Verification items for the finished model (mm, model axes). A direction names the side the tool comes from. Give positions to 0.01 mm unless a question says otherwise; leave off trailing zeros. Loops run counter-clockwise (first coordinate to the right, second up) from the corner with the lowest first, then second, coordinate; pieces in that order, holes last. Notation, with made-up numbers: (29.25, -19) - (55.25, -19) arc R35 cw to (55.25, 17) - close; hole circle Ø1 at (86, 35). An arc over 180 degrees is marked (long way). Put each result on its own line as item: value. Start each with the question number.
```python
from build123d import *

# Parameters (mm, degrees)
SKETCH1_W                                           = 8
SKETCH1_H                                           = 105
BASE_DEPTH                                          = 35
CSK_FOR_M4_COUNTERSUNK_FLAT_HEAD_SCREW2_D           = 4.5
CSK_FOR_M4_COUNTERSUNK_FLAT_HEAD_SCREW2_CSINK_D     = 9.4
CSK_FOR_M4_COUNTERSUNK_FLAT_HEAD_SCREW2_CSINK_ANGLE = 90
FILLET1_R                                           = 35
SKETCH8_W                                           = 8
SKETCH8_H                                           = 70
BOSS_EXTRUDE1_DEPTH                                 = 101.6
CUT_EXTRUDE1_REACH                                  = 112.968
CUT_EXTRUDE2_DEPTH                                  = 111.968463989
FILLET2_R                                           = 34.925
FILLET3_R                                           = 15.875
SKETCH12_R                                          = 12.7
CUT_EXTRUDE4_DEPTH                                  = 111.968463989
CHAMFER1_SIZE                                       = 0.396875


with BuildPart() as part:
    # Sketch1 → base (new, symmetric)
    with BuildSketch(Plane.XY):
        with Locations((4, 52.5)):
            Rectangle(SKETCH1_W, SKETCH1_H)
    extrude(amount=BASE_DEPTH, both=True)

    # CSK for M4 Countersunk Flat Head Screw2 (through all)
    with Locations(Plane.ZY):
        with Locations((-11.125, 50.730934766), (-22.25, 70), (-11.125, 89.269065234), (11.125, 89.269065234), (22.25, 70), (11.125, 50.730934766)):
            CounterSinkHole(CSK_FOR_M4_COUNTERSUNK_FLAT_HEAD_SCREW2_D / 2, CSK_FOR_M4_COUNTERSUNK_FLAT_HEAD_SCREW2_CSINK_D / 2, counter_sink_angle=CSK_FOR_M4_COUNTERSUNK_FLAT_HEAD_SCREW2_CSINK_ANGLE)

    # Fillet1
    fillet1_edges = [part.edges().sort_by_distance(p)[0] for p in [
        (4, 105, 35),
        (4, 105, -35),
    ]]
    fillet(fillet1_edges, radius=FILLET1_R - 0.0001)  # a hair under: the kernel refuses the full size

    # Sketch8 → Boss-Extrude1 (add)
    with BuildSketch(Plane.XZ):
        with Locations((4, 0)):
            Rectangle(SKETCH8_W, SKETCH8_H)
    extrude(amount=BOSS_EXTRUDE1_DEPTH)

    # Sketch9 → Cut-Extrude1 (cut, up to next)
    with BuildSketch(Plane.ZY, mode=Mode.PRIVATE) as cut_extrude1_sk1:
        with BuildLine():
            Line((2.5, 22.225), (2.5, -85.725))
            ThreePointArc((2.5, -85.725), (0, -88.225), (-2.5, -85.725))
            Line((-2.5, -85.725), (-2.5, 22.225))
            ThreePointArc((-2.5, 22.225), (0, 24.725), (2.5, 22.225))
        make_face()
    cut_extrude1_tool1 = extrude(cut_extrude1_sk1.sketch, amount=-CUT_EXTRUDE1_REACH, mode=Mode.PRIVATE) & part.part
    add(cut_extrude1_tool1.solids().sort_by_distance((0, -31.75, 0))[0], mode=Mode.SUBTRACT)

    # Sketch10 → Cut-Extrude2 (cut, through all)
    with BuildSketch(Plane(origin=(8, 0, 0), x_dir=(0, 0, -1), z_dir=(1, 0, 0))):
        with BuildLine():
            Line((15.875, 38.807302537), (15.875, -101.6))
            Line((15.875, -101.6), (35, -101.6))
            Line((35, -101.6), (35, 70))
            ThreePointArc((35, 70), (29.838104833, 51.705533624), (15.875, 38.807302537))
        make_face()
        with BuildLine():
            Line((-35, -101.6), (-15.875, -101.6))
            Line((-15.875, -101.6), (-15.875, 38.807302537))
            ThreePointArc((-15.875, 38.807302537), (-29.838104833, 51.705533624), (-35, 70))
            Line((-35, 70), (-35, -101.6))
        make_face()
    extrude(amount=-CUT_EXTRUDE2_DEPTH, mode=Mode.SUBTRACT)

    # Fillet2
    fillet2_edges = [part.edges().sort_by_distance(p)[0] for p in [
        (4, 38.807302537, -15.875),
        (4, 38.807302537, 15.875),
    ]]
    fillet(fillet2_edges, radius=FILLET2_R)

    # Fillet3
    fillet3_edges = [part.edges().sort_by_distance(p)[0] for p in [
        (4, -101.6, -15.875),
        (4, -101.6, 15.875),
    ]]
    fillet(fillet3_edges, radius=FILLET3_R - 0.0001)  # a hair under: the kernel refuses the full size

    # Sketch12 → Cut-Extrude4 (cut, through all)
    with BuildSketch(Plane.ZY):
        with Locations(Location((0, 70, 0), (0, 0, 270))):
            Circle(SKETCH12_R)
    extrude(amount=-CUT_EXTRUDE4_DEPTH, mode=Mode.SUBTRACT)

    # Chamfer1
    chamfer1_edges = [part.edges().sort_by_distance(p)[0] for p in [
        (8, 94.748766631, -24.748766631),
        (0, 94.748766631, 24.748766631),
        (8, 34.864684854, -18.350815522),
        (0, 34.864684854, -18.350815522),
        (8, 34.864684854, 18.350815522),
        (0, 34.864684854, 18.350815522),
        (8, -31.887878432, -15.875),
        (8, -31.887878432, 15.875),
        (8, -96.950349441, 11.225349441),
        (8, -96.950349441, -11.225349441),
        (0, -31.887878432, -15.875),
        (0, -31.887878432, 15.875),
        (0, -96.950349441, 11.225349441),
        (0, -96.950349441, -11.225349441),
        (8, 82.7, 0),
        (0, 82.7, 0),
        (0, 94.748766631, -24.748766631),
        (8, 94.748766631, 24.748766631),
        (0, 24.725, 0),
        (0, -31.75, -2.5),
        (0, -88.225, 0),
        (0, -31.75, 2.5),
        (8, -31.75, -2.5),
        (8, 24.725, 0),
        (8, -31.75, 2.5),
        (8, -88.225, 0),
    ]]
    chamfer(chamfer1_edges, length=CHAMFER1_SIZE)


solid = part.part
```
1) Section check A-A, the plane y = -42. Enter the section's corners in (x, z) (3 decimals).
2) Draft check along Z on faces 4 (the face through (3.95, -88.224, 0.055)), 5 (the face through (4, -33, 15.875)), 6 (the face through (3.95, -96.826, -11.348)). Enter one of: pulls with the +Z half, pulls with the -Z half, needs draft (parallel to the pull), parting line crosses it, or undercut.
3) Section check B-B, the plane x = 5. State how many separate pieces and enclosed holes the cut face has, plus the area to 3 significant figures.
4) Set-up check for faces 1 (the face through (4, -31, -15.875)), 2 (the face through (7.893, 94.813, -24.273)), 3 (the face through (3.95, 24.724, -0.055)): record each of +Z, -Z, +X, -X, +Y, -Y from which the full face is reachable in a straight line by a thin tool's end or side.
5) Scan lines: line 1 along Z through (x, y) = (6.1, 70); line 2 along Z through (x, y) = (7, 2) (3 decimals); line 3 along Y through (x, z) = (5, -10.5). Record each from-to range of solid material in increasing order. Write a range as from..to.
6) Depth check by flat-ended pin: P1, Ø3.5, axis at x = 4, y = -41, coming from the -Z side (3 decimals); P2, Ø1.5, axis at x = 1.5, z = 8, coming from the -Y side; P3, Ø1.5, axis at x = 6.5, z = 10.5, coming from the -Y side. Enter the tip coordinate at first touch or a pass-through.
Results are:
1. outline: (0, -15.478) - (0.397, -15.875) - (7.603, -15.875) - (8, -15.478) - (8, -2.897) - (7.603, -2.5) - (0.397, -2.5) - (0, -2.897) - close; (0, 2.897) - (0.397, 2.5) - (7.603, 2.5) - (8, 2.897) - (8, 15.478) - (7.603, 15.875) - (0.397, 15.875) - (0, 15.478) - close
2. face 4: undercut
2. face 5: pulls with the +Z half
2. face 6: pulls with the -Z half
3. separate pieces: 1
3. enclosed holes: 8
3. area: 7,020 mm2
4. face 1: -Z, +X, -X, -Y
4. face 2: -Z, +X, +Y
4. face 3: +X, -X
5. line 1: z = -35..-24.5, -20..-12.7, 12.7..20, 24.5..35
5. line 2: z = -15.875..-2.5, 2.5..15.875
5. line 3: y = -97.63..48.57, 52.89..62.86, 77.14..87.11, 91.43..103.39
6. P1: stops at z = -15.875
6. P2: stops at y = -99.85
6. P3: stops at y = -98.25
